Geometry: see drawing. Coordinates: mm, zero at the bounding-box minimum. A direction names the side the tool comes from. Coordinates: 2 decimals unless noted, no trailing zeros. Write each loop counter-clockwise with the first axis right and the second up, starting at its lowest first coordinate (ties: lowest second). Pieces come first, ordered by that corner, then holes.
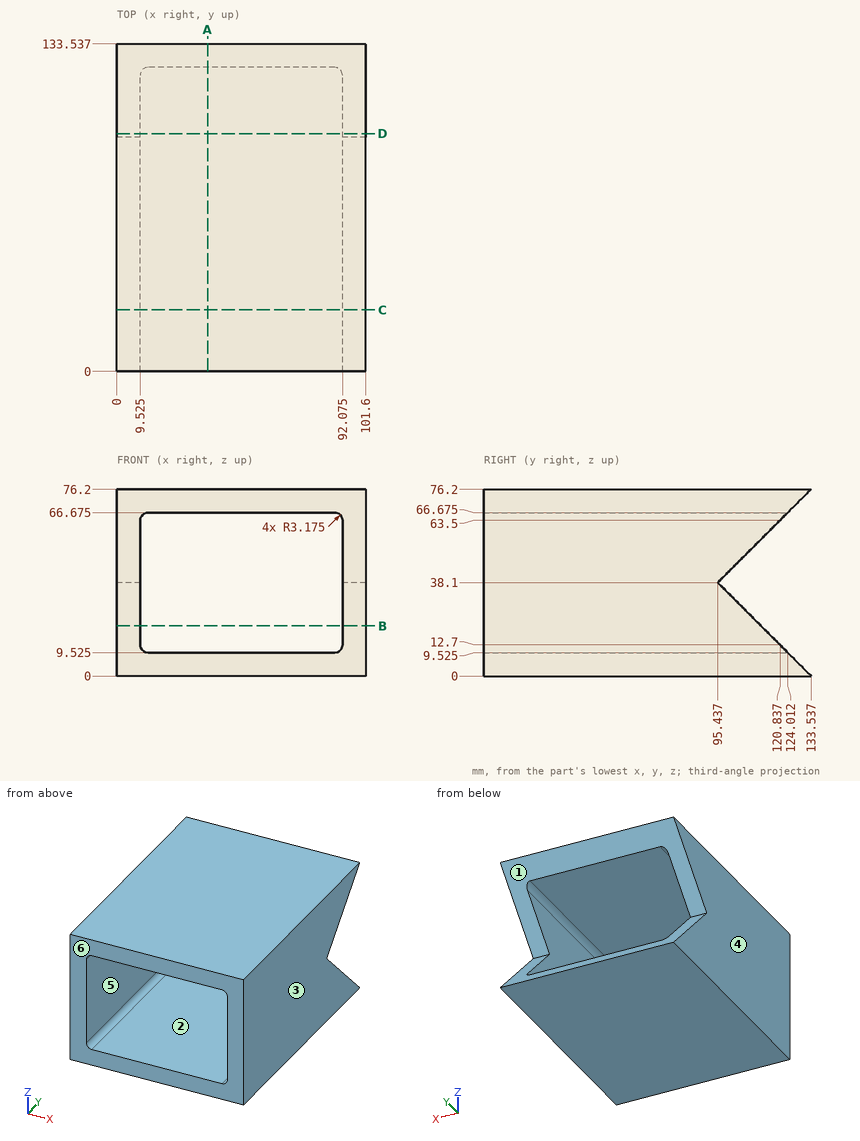
Item 1: Material intervals for probe 1 along Z at (x, y) = (88.5, 11.5) (3 decimals); probe 2 along X at (y, z) = (82.5, 16) (3 decimals); probe 3 along X at (y, z) = (67.5, 65), sorted ascending.
Derived:
probe 1: z = 0 to 9.525, 66.675 to 76.2
probe 2: x = 0 to 9.525, 92.075 to 101.6
probe 3: x = 0 to 9.9, 91.7 to 101.6
Item 2: Section D-D, the plane y = 97. Output: boundary loops of the cut face in (x, z) (3 decimals), plus the area to 3 significant figures.
Derived:
outline: (0, 0) - (101.6, 0) - (101.6, 36.537) - (92.075, 36.537) - (92.075, 12.7) arc R3.175 cw to (88.9, 9.525) - (12.7, 9.525) arc R3.175 cw to (9.525, 12.7) - (9.525, 36.537) - (0, 36.537) - close; (0, 39.663) - (9.525, 39.663) - (9.525, 63.5) arc R3.175 cw to (12.7, 66.675) - (88.9, 66.675) arc R3.175 cw to (92.075, 63.5) - (92.075, 39.663) - (101.6, 39.663) - (101.6, 76.2) - (0, 76.2) - close
area: 2,970 mm2
Item 3: Set-up query: the marked faces 5 and 6. Return all of +Z, -Z, +X, -X, +Y, -Y with unobstructed straight access to the full face (end or side cutting, diameter ignored); none if empty.
Derived:
face 5: +Y, -Y
face 6: +Z, -Z, +X, -X, -Y
Item 4: Section C-C, the plane y = 25. Output: boundary loops of the cut face in (x, z) (3 decimals).
Derived:
outline: (0, 0) - (101.6, 0) - (101.6, 76.2) - (0, 76.2) - close; hole (9.525, 12.7) arc R3.175 ccw to (12.7, 9.525) - (88.9, 9.525) arc R3.175 ccw to (92.075, 12.7) - (92.075, 63.5) arc R3.175 ccw to (88.9, 66.675) - (12.7, 66.675) arc R3.175 ccw to (9.525, 63.5) - close
Item 5: Section A-A, the plane x = 37. Output: boundary loops of the cut face in (y, z) (3 decimals).
Derived:
outline: (0, 0) - (133.537, 0) - (124.012, 9.525) - (0, 9.525) - close; (0, 66.675) - (124.012, 66.675) - (133.537, 76.2) - (0, 76.2) - close
Item 6: Pin query (flat end, axial travel): pin 1 (8 mm diameter, centred on x = 87, z = 63, fed in from +Y); pin 2 (8 mm diameter, centred on y = 20.5, z = 14, fed in from -X). Return the tip coordinate at first contact, or that it passes through.
Derived:
pin 1: stops at y = 124.34
pin 2: stops at x = 0
Item 7: Pull-direction query (X, two-part tool) for the marked faces 1, 2, 3 and 4; classes: released by +X, released by -X, zero draft, split by the parting line, or undercut.
Derived:
face 1: zero draft
face 2: undercut
face 3: released by +X
face 4: released by -X
Item 8: Section B-B, the plane z = 20.5. Output: boundary loops of the cut face in (x, y) (3 decimals).
Derived:
outline: (0, 0) - (9.525, 0) - (9.525, 113.037) - (0, 113.037) - close; (92.075, 0) - (101.6, 0) - (101.6, 113.037) - (92.075, 113.037) - close
